The model under review builds one solid part; all positions refer to its coordinate system, in mm. Face numbers are marked on the shaded views. A direction names the side the tool comes from. Round coordinates to 2 decimals unless told otherwise and drop trailing zeros. Order: outer loops, then holes, each group sorted by start corner. A loop starts at its lowest first (then second) coordinate and runs counter-clockwise, first axis right, second up. Notation, with made-up numbers: M -6,23.5 L 4,23.5 A14 ccw 4,41.5 Z; hole C 16.5,-34.75 d11. An arc over 180 degrees is marked long. Use a Markdown table: item, result. Add a question column.
1. For the marked faces 1 and 2, list the 3-axis set-ups (+Z, -Z, +X, -X, +Y, -Y) from which the entire face can be reached by the end or side of a thin tool; tool diameter is ignored.
2. Consider section C-C on y = 2. State the section outline as (x, z) points, then the cut area to 3 significant figures.
3. The part is to be moulded in two halves that separate along X. For the marked faces 3, 4 and 5, say which applies: +X half, -X half, draft (parallel to the pull), parting line (faces both ways), or undercut.
4. To check wall thickness, follow probe 1 along Z at (x, y) = (0.5, 2); probe 2 along Z at (x, y) = (73.5, 4.5); probe 3 along Y at (x, z) = (82, 19.5). State the ranges of each line that lie inside material, in increasing order.
5. Consider section A-A on z = 8. State the section outline as (x, y) points.
6. Consider section B-B on x = 62. Count the separate pieces of the cut face and the enclosed holes in it, then the cut area to 3 significant figures.
7. Insertion check: P1, Ø6, axis at y = 34, z = 41.5, coming from the +X side; P2, Ø1.6, axis at y = -0.5, z = 74.5, coming from the +X side; P3, Ø1, axis at y = 5, z = 67.5, coming from the +X side. Each pin has a flat end and moves straight along its axis. Give the tip position at first contact, or say it passes through.
8. Consider section D-D on z = 58.5. State the section outline as (x, y) points.
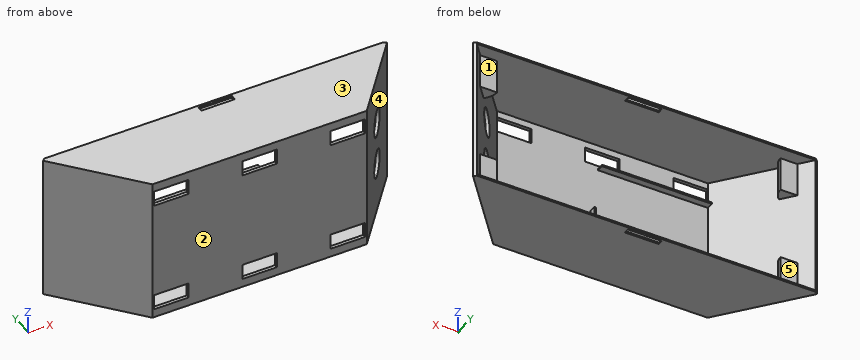
from build123d import *

# Parameters (mm, degrees)
EXTRU_MINCE1_DEPTH      = 85
BOSS_EXTRU_1_DEPTH      = 1
BOSS_EXTRU_2_DEPTH      = 1
ESQUISSE7_W             = 20
ESQUISSE7_H             = 10
R_VOL_MINCE1_ANGLE      = 50
ESQUISSE8_W             = 20
ESQUISSE8_H             = 10
R_VOL_MINCE2_ANGLE      = 50
ESQUISSE9_W             = 20
ESQUISSE9_H             = 10
R_VOL_MINCE3_ANGLE      = 50
ESQUISSE10_W            = 20
ESQUISSE10_H            = 10
R_VOL_MINCE4_ANGLE      = 50
ESQUISSE12_W            = 20.5
ESQUISSE12_H            = 9
ENL_V_MAT_EXTRU_2_DEPTH = 10
ESQUISSE13_W            = 20.5
ESQUISSE13_H            = 9
ENL_V_MAT_EXTRU_3_DEPTH = 10
ESQUISSE14_W            = 65
ESQUISSE14_H            = 1
EXTRU_MINCE2_DEPTH      = 4
ESQUISSE15_W            = 1
ESQUISSE15_H            = 10
EXTRU_MINCE3_DEPTH      = 4
ESQUISSE16_W            = 20
ESQUISSE16_H            = 3
ENL_V_MAT_EXTRU_4_DEPTH = 10
ESQUISSE17_W            = 20
ESQUISSE17_H            = 3
ENL_V_MAT_EXTRU_5_DEPTH = 10
ESQUISSE19_R            = 8.005
ENL_V_MAT_EXTRU_6_DEPTH = 10


with BuildPart() as part:
    # Esquisse3 → Extru.-Mince1 (new body)
    with BuildSketch(Plane.XY):
        Polygon((-37.759483403, 45), (0, 0), (125, 0), (162.759483403, 45), (164.291572289, 43.714424781), (125.932615316, -2), (-0.932615316, -2), (-39.291572289, 43.714424781), align=None)
    extrude(amount=EXTRU_MINCE1_DEPTH)

    # Esquisse5 → Boss.-Extru.1 (add)
    with BuildSketch(Plane(origin=(0, 0, 0), x_dir=(-1, 0, 0), z_dir=(0, 0, -1))):
        Polygon((-162.759483403, 45), (37.759483403, 45), (0, 0), (-125, 0), align=None)
    extrude(amount=-BOSS_EXTRU_1_DEPTH)

    # Esquisse6 → Boss.-Extru.2 (add)
    with BuildSketch(Plane.XY.offset(85)):
        Polygon((162.759483403, 45), (-37.759483403, 45), (0, 0), (125, 0), align=None)
    extrude(amount=-BOSS_EXTRU_2_DEPTH)

    # Esquisse7 → Révol.-Mince1 (revolve)
    with BuildSketch(Plane(origin=(0, 0, 0), x_dir=(0, 0, -1), z_dir=(0.7660444431189791, 0.642787609686538, 0))):
        with Locations((-74, 43.74332802)):
            Rectangle(ESQUISSE7_W, ESQUISSE7_H)
    revolve(axis=Axis((-31.331607306, 37.339555569, 84), (0, 0, 1)), revolution_arc=R_VOL_MINCE1_ANGLE)

    # Esquisse8 → Révol.-Mince2 (revolve)
    with BuildSketch(Plane(origin=(0, 0, 0), x_dir=(0, 0, -1), z_dir=(0.7660444431189791, 0.642787609686538, 0))):
        with Locations((-11, 43.74332802)):
            Rectangle(ESQUISSE8_W, ESQUISSE8_H)
    revolve(axis=Axis((-31.331607306, 37.339555569, 1), (0, 0, 1)), revolution_arc=R_VOL_MINCE2_ANGLE)

    # Esquisse9 → Révol.-Mince3 (revolve)
    with BuildSketch(Plane(origin=(73.353011104, -61.550484563, 0), x_dir=(0, 0, 1), z_dir=(-0.7660444431189796, 0.6427876096865375, 0))):
        with Locations((74, 124.091779231)):
            Rectangle(ESQUISSE9_W, ESQUISSE9_H)
    revolve(axis=Axis((156.331607306, 37.339555569, 84), (0, 0, -1)), revolution_arc=R_VOL_MINCE3_ANGLE)

    # Esquisse10 → Révol.-Mince4 (revolve)
    with BuildSketch(Plane(origin=(73.353011104, -61.550484563, 0), x_dir=(0, 0, 1), z_dir=(-0.7660444431189796, 0.6427876096865375, 0))):
        with Locations((11, 124.091779231)):
            Rectangle(ESQUISSE10_W, ESQUISSE10_H)
    revolve(axis=Axis((156.331607306, 37.339555569, 1), (0, 0, -1)), revolution_arc=R_VOL_MINCE4_ANGLE)

    # Esquisse12 → Enlèv. mat.-Extru.2 (cut)
    with BuildSketch(Plane(origin=(0, 0, 0), x_dir=(1, 0, 0), z_dir=(0, 1, 0))):
        with Locations((10.25, -9.5)):
            Rectangle(ESQUISSE12_W, ESQUISSE12_H)
        with Locations((10.25, -75.5)):
            Rectangle(ESQUISSE12_W, ESQUISSE12_H)
        with Locations((114.75, -9.5)):
            Rectangle(ESQUISSE12_W, ESQUISSE12_H)
        with Locations((114.75, -75.5)):
            Rectangle(ESQUISSE12_W, ESQUISSE12_H)
    extrude(amount=-ENL_V_MAT_EXTRU_2_DEPTH, mode=Mode.SUBTRACT)

    # Esquisse13 → Enlèv. mat.-Extru.3 (cut)
    with BuildSketch(Plane(origin=(0, 0, 0), x_dir=(1, 0, 0), z_dir=(0, 1, 0))):
        with Locations((62.5, -9.5)):
            Rectangle(ESQUISSE13_W, ESQUISSE13_H)
        with Locations((62.5, -75.5)):
            Rectangle(ESQUISSE13_W, ESQUISSE13_H)
    extrude(amount=-ENL_V_MAT_EXTRU_3_DEPTH, mode=Mode.SUBTRACT)

    # Esquisse14 → Extru.-Mince2 (add)
    with BuildSketch(Plane(origin=(0, 0, 0), x_dir=(1, 0, 0), z_dir=(0, 1, 0))):
        with Locations((32.5, -15.319657918)):
            Rectangle(ESQUISSE14_W, ESQUISSE14_H)
        with Locations((32.5, -68.819657918)):
            Rectangle(ESQUISSE14_W, ESQUISSE14_H)
    extrude(amount=EXTRU_MINCE2_DEPTH)

    # Esquisse15 → Extru.-Mince3 (add)
    with BuildSketch(Plane(origin=(0, 0, 0), x_dir=(1, 0, 0), z_dir=(0, 1, 0))):
        with Locations((69, -35.819657918)):
            Rectangle(ESQUISSE15_W, ESQUISSE15_H)
    extrude(amount=EXTRU_MINCE3_DEPTH)

    # Esquisse16 → Enlèv. mat.-Extru.4 (cut)
    with BuildSketch(Plane.XY.offset(1)):
        with Locations((62.5, 42)):
            Rectangle(ESQUISSE16_W, ESQUISSE16_H)
    extrude(amount=-ENL_V_MAT_EXTRU_4_DEPTH, mode=Mode.SUBTRACT)

    # Esquisse17 → Enlèv. mat.-Extru.5 (cut)
    with BuildSketch(Plane(origin=(0, 0, 84), x_dir=(-1, 0, 0), z_dir=(0, 0, -1))):
        with Locations((-62.5, 42)):
            Rectangle(ESQUISSE17_W, ESQUISSE17_H)
    extrude(amount=-ENL_V_MAT_EXTRU_5_DEPTH, mode=Mode.SUBTRACT)

    # Esquisse19 → Enlèv. mat.-Extru.6 (cut)
    with BuildSketch(Plane(origin=(74.88509999, -62.836059783, 0), x_dir=(0, 0, -1), z_dir=(0.7660444431189799, -0.6427876096865373, 0))):
        with Locations(Location((-29.5, 109.415835895, 0), (0, 0, 90))):
            Circle(ESQUISSE19_R)
        with Locations(Location((-55.5, 109.415835895, 0), (0, 0, 90))):
            Circle(ESQUISSE19_R)
    extrude(amount=-ENL_V_MAT_EXTRU_6_DEPTH, mode=Mode.SUBTRACT)


solid = part.part
Answer block:
| question | item | result |
|---|---|---|
| 1 | face 1 | +Y |
| 1 | face 2 | +Z, -Z, +X, -X, -Y |
| 2 | outline | M -4.29,0 L 129.29,0 L 129.29,85 L -4.29,85 Z; M 0,14.82 L 65,14.82 L 65,15.82 L 0,15.82 Z; M 0,68.32 L 65,68.32 L 65,69.32 L 0,69.32 Z; M 68.5,30.82 L 69.5,30.82 L 69.5,40.82 L 68.5,40.82 Z; hole M -1.68,1 L 126.68,1 L 126.68,84 L -1.68,84 Z |
| 2 | area | 841 mm^2 |
| 3 | face 3 | draft |
| 3 | face 4 | +X half |
| 3 | face 5 | undercut |
| 4 | probe 1 | 0 to 1, 14.82 to 15.82, 68.32 to 69.32, 84 to 85 |
| 4 | probe 2 | 0 to 1, 84 to 85 |
| 4 | probe 3 | -2 to 0 |
| 5 | outline | M -39.29,43.71 L -0.93,-2 L 0,-2 L 0,0 L -24.9,29.68 A10 ccw -21.33,37.34 L -31.33,37.34 L -37.76,45 Z; M 20.5,-2 L 52.25,-2 L 52.25,0 L 20.5,0 Z; M 72.75,-2 L 104.5,-2 L 104.5,0 L 72.75,0 Z; M 125,-2 L 125.93,-2 L 164.29,43.71 L 162.76,45 L 156.33,37.34 L 146.33,37.34 A10 ccw 149.9,29.68 L 125,0 Z |
| 6 | separate pieces | 5 |
| 6 | enclosed holes | 0 |
| 6 | area | 226 mm^2 |
| 7 | P1 | x = 158.66 |
| 7 | P2 | x = 127.86 |
| 7 | P3 | x = 132.23 |
| 8 | outline | M -39.29,43.71 L -0.93,-2 L 125.93,-2 L 140.45,15.3 L 138.91,16.58 L 125,0 L 0,0 L -37.76,45 Z; M 148.45,27.95 L 149.99,26.67 L 164.29,43.71 L 162.76,45 Z |
